Work out the finished part from the listing and answer in its coordinate system (mm). A direction names the side the tool comes from. Coordinates: 2 decimals unless noted, no trailing zeros. Loops run counter-clockwise (first coordinate to the right, second up) from the corner with the lowest first, then second, coordinate; pieces in that order, holes last. Notation, with made-up numbers: (72, 36.5) - (109, 36.5) arc R32 ccw to (109, 63.5) - close; hole circle Ø4 at (84, 61). An arc over 180 degrees is marked (long way). Write each question's results on one line, items separated by ' | '. Start each with the question number.
Item 1: Section B-B, the plane y = 0.25 is taken. Write down the section's boundary in (x, z) (3 decimals).
Item 2: For a pull along X with two mould halves and no side action, classify faces 1 (the face through (25.4, 0, 341)), 2 (the face through (22.225, 0, 344)), 3 (the face through (0, -9.525, 359)), 4 (the face through (0, 12.7, 365)) as +X half, -X half, draft (parallel to the pull), parting line (faces both ways), or undercut.
Item 3: Section C-C, the plane x = -3 is taken. Write down the section's boundary in (y, z) (3 decimals), plus the area to 3 significant figures.
Item 4: Section A-A, the plane z = 286 is taken. Write down the section's boundary in (x, y) (3 decimals), plus the area to 3 significant figures.
Item 5: A tool of negligible diameter and unlimited length cuts with its end or side. For faces 5 (the face through (0, 9.525, 365)), 6 (the face through (7.661, -10.407, 698.646)), from which of +Z, -Z, +X, -X, +Y, -Y can it reach the whole face along a straight path? Write none if from no direction.
Item 6: Consider probe 1 along X at (y, z) = (-4.5, 574.5) (3 decimals); probe 2 along Y at (x, z) = (11.5, 334.5) (3 decimals); probe 3 along Z at (x, y) = (-16, -10.5). Determine where each line is inside the solid, lowest interval first. Write a range as [from, to].
from build123d import *

# Parameters (mm, degrees)
SKETCH1_W                = 50.8
SKETCH1_H                = 25.4
SKETCH1_W_2              = 44.45
SKETCH1_H_2              = 19.05
BOSS_EXTRUDE1_DEPTH      = 771.9314
CUT_EXTRUDE1_DEPTH       = 773.76672179
SKETCH10_W               = 90.356784756
SKETCH10_H               = 129.906903396
CUT_EXTRUDE8_DEPTH       = 40.64
CUT_EXTRUDE9_DEPTH       = 1230.239509376
CUT_EXTRUDE10_DEPTH      = 567.92953801
CUT_EXTRUDE10_DEPTH_BACK = 567.92953801


with BuildPart() as part:
    # Sketch1 → Boss-Extrude1 (new body)
    with BuildSketch(Plane.XY):
        Rectangle(SKETCH1_W, SKETCH1_H)
        Rectangle(SKETCH1_W_2, SKETCH1_H_2, mode=Mode.SUBTRACT)
    extrude(amount=BOSS_EXTRUDE1_DEPTH)

    # Sketch2 → Cut-Extrude1 (cut, through all)
    with BuildSketch(Plane(origin=(0, 12.7, 0), x_dir=(1, 0, 0), z_dir=(0, 1, 0))):
        Polygon((25.4, 0), (-25.4, -50.8), (-25.4, 0), align=None)
        Polygon((-25.4, -771.9314), (25.4, -721.1314), (25.4, -771.9314), align=None)
    extrude(amount=-CUT_EXTRUDE1_DEPTH, mode=Mode.SUBTRACT)

    # Sketch10 → Cut-Extrude8 (cut)
    with BuildSketch(Plane(origin=(-369.87845504, 0, 369.87845504), x_dir=(-0.7071067811865528, 0, -0.7071067811865422), z_dir=(0.7071067811865422, 0, -0.7071067811865528))):
        with Locations((-494.442187508, 23.675993241)):
            Rectangle(SKETCH10_W, SKETCH10_H)
    extrude(amount=-CUT_EXTRUDE8_DEPTH, mode=Mode.SUBTRACT)


with BuildPart() as cut_extrude8_piece_1:
    # of the separate pieces the step leaves, piece 1, a body of its own (cut_extrude8_pieces)
    add(part.part.solids().sort_by_distance((25.4, -12.7, 0))[0])

    # Sketch11 → Cut-Extrude9 (cut, through all)
    with BuildSketch(Plane(origin=(386.259110354, 0, -386.259110354), x_dir=(-0.7071067811865541, -3.472433466129024e-15, -0.7071067811865409), z_dir=(0.7071067811865409, -3.4724334661290888e-15, -0.7071067811865541))):
        Polygon((-17.960512242, -12.7), (-26.213472526, 12.7), (-17.960512242, 12.7), align=None)
    extrude(amount=-CUT_EXTRUDE9_DEPTH, mode=Mode.SUBTRACT)


with BuildPart() as cut_extrude8_piece_2:
    # of the separate pieces the step leaves, piece 2, a body of its own (cut_extrude8_pieces)
    add(part.part.solids().sort_by_distance((-25.349574627, -12.7, 771.880974627))[0])


with BuildPart() as cut_extrude10_tool:
    # Sketch12 → Cut-Extrude10 (new, two sides: drawn at the far end of the back side and taken through both)
    with BuildSketch(Plane(origin=(-332.161379331, 0, 332.161379331), x_dir=(-0.7071067811865526, 0, -0.7071067811865425), z_dir=(0.7071067811865425, 0, -0.7071067811865526)).offset(-CUT_EXTRUDE10_DEPTH_BACK)):
        Polygon((-498.689041164, -12.7), (-506.942001448, 12.7), (-527.877415309, 12.7), (-527.877415309, -12.7), align=None)
    extrude(amount=CUT_EXTRUDE10_DEPTH + CUT_EXTRUDE10_DEPTH_BACK)


with BuildPart() as cut_extrude8_piece_1_1:
    add(cut_extrude8_piece_1.part)

    # Cut-Extrude10: cut by cut_extrude10_tool
    add(cut_extrude10_tool.part, mode=Mode.SUBTRACT)


with BuildPart() as cut_extrude8_piece_2_1:
    add(cut_extrude8_piece_2.part)

    # Cut-Extrude10: cut by cut_extrude10_tool
    add(cut_extrude10_tool.part, mode=Mode.SUBTRACT)


solid = cut_extrude8_piece_1_1.part
Answer key:
1) outline: (-25.4, 56.751) - (-22.225, 53.576) - (-22.225, 717.532) - (-25.4, 714.357) - close; (22.225, 9.126) - (25.4, 5.951) - (25.4, 685.803) - (22.225, 688.978) - close
2) face 1: +X half | face 2: undercut | face 3: undercut | face 4: draft
3) outline: (-12.7, 28.4) - (-9.525, 29.859) - (-9.525, 709.712) - (-12.7, 708.253) - close; (9.525, 38.613) - (12.7, 40.071) - (12.7, 719.924) - (9.525, 718.465) - close | area: 4,320 mm^2
4) outline: (-25.4, -12.7) - (25.4, -12.7) - (25.4, 12.7) - (-25.4, 12.7) - close; hole (-22.225, -9.525) - (22.225, -9.525) - (22.225, 9.525) - (-22.225, 9.525) - close | area: 444 mm^2
5) face 5: +Z, -Z | face 6: +Z, +X, -Y
6) probe 1: x = [-25.4, -22.225], [22.225, 25.4] | probe 2: y = [-12.7, -9.525], [9.525, 12.7] | probe 3: z = [42.41, 722.26]
